Build history of the part. All positions in model axes, mm. Face numbers are marked on the shaded views. A direction names the side the tool comes from. Coordinates: 2 decimals unless noted, no trailing zeros. Order: outer loops, then holes, each group sorted by start corner. A loop starts at its lowest first (then second) coordinate and runs counter-clockwise, first axis right, second up. Notation, with made-up numbers: (71.5, 30) - (100.5, 30) arc R15 ccw to (100.5, 44) - close; hole circle Ø1 at (-11, 82.5). An arc over 180 degrees is marked (long way). Write each question's results on one line, items separated by ' | '. Start each with the question number.
Autodesk Fusion 360 part; units mm, degrees
sketch "Sketch1" plane through (0, 0, 0) normal (0, 0, 1) x (1, 0, 0)
  circle A0 centre (0, 0) radius 3.55
  dimension "d1" = 7.1
extrude "Extrude1" add sketch "Sketch1" along normal blind 16
hole "Hole1" at (0, 0, 16) direction (0, 0, -1) diameter 4.7 depth 5 tip angle 180
hole "Hole2" at (0, 0, 0) direction (0, 0, 1) diameter 4.7 depth 5 tip angle 180
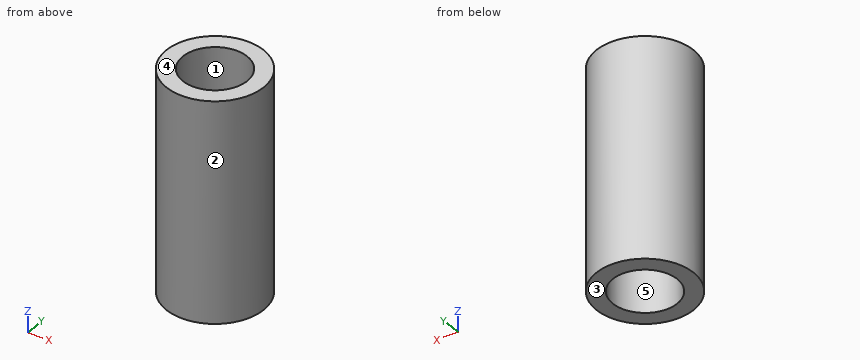
Item 1: Slice it at C-C (z = 12.5). Write the cut outline in (x, y), then the cut area to 3 significant figures.
Item 2: Probe probe 1 along Y at (x, z) = (0, 3.95); probe 2 along Z at (x, y) = (-2, 0.75); probe 3 along Y at (x, z) = (-2, 15.5). List the from-to ranges inside material, lowest first.
Item 3: Slice it at D-D (y = -2.75). Write the cut outline in (x, z) (3 decimals), then the cut area to 3 significant figures.
Item 4: Which spindle directions (+Z, -Z, +X, -X, +Y, -Y) get a long thin tool onto all of the face, cutting with end or side? Do the marked faces 4 and 5. Say none if no direction does.
Item 5: Slice it at A-A (x = 0). Write the cut outline in (y, z), then the cut area to 3 significant figures.
Item 6: Pull direction Y, two halves, no side cores. Call the marked faces 1, 2 and 3: released by +Y, released by -Y, zero draft, split by the parting line, or undercut.
Resolved:
1) outline: circle Ø7.1 at (0, 0); hole circle Ø4.7 at (0, 0) | area: 22.2 mm^2
2) probe 1: -3.55 to -2.35, 2.35 to 3.55 | probe 2: 5 to 11 | probe 3: -2.93 to -1.23, 1.23 to 2.93
3) outline: (-2.245, 0) - (2.245, 0) - (2.245, 16) - (-2.245, 16) - close | area: 71.8 mm^2
4) face 4: +Z, +X, -X, +Y, -Y | face 5: -Z
5) outline: (-3.55, 0) - (-2.35, 0) - (-2.35, 5) - (2.35, 5) - (2.35, 0) - (3.55, 0) - (3.55, 16) - (2.35, 16) - (2.35, 11) - (-2.35, 11) - (-2.35, 16) - (-3.55, 16) - close | area: 66.6 mm^2
6) face 1: undercut | face 2: split by the parting line | face 3: zero draft
